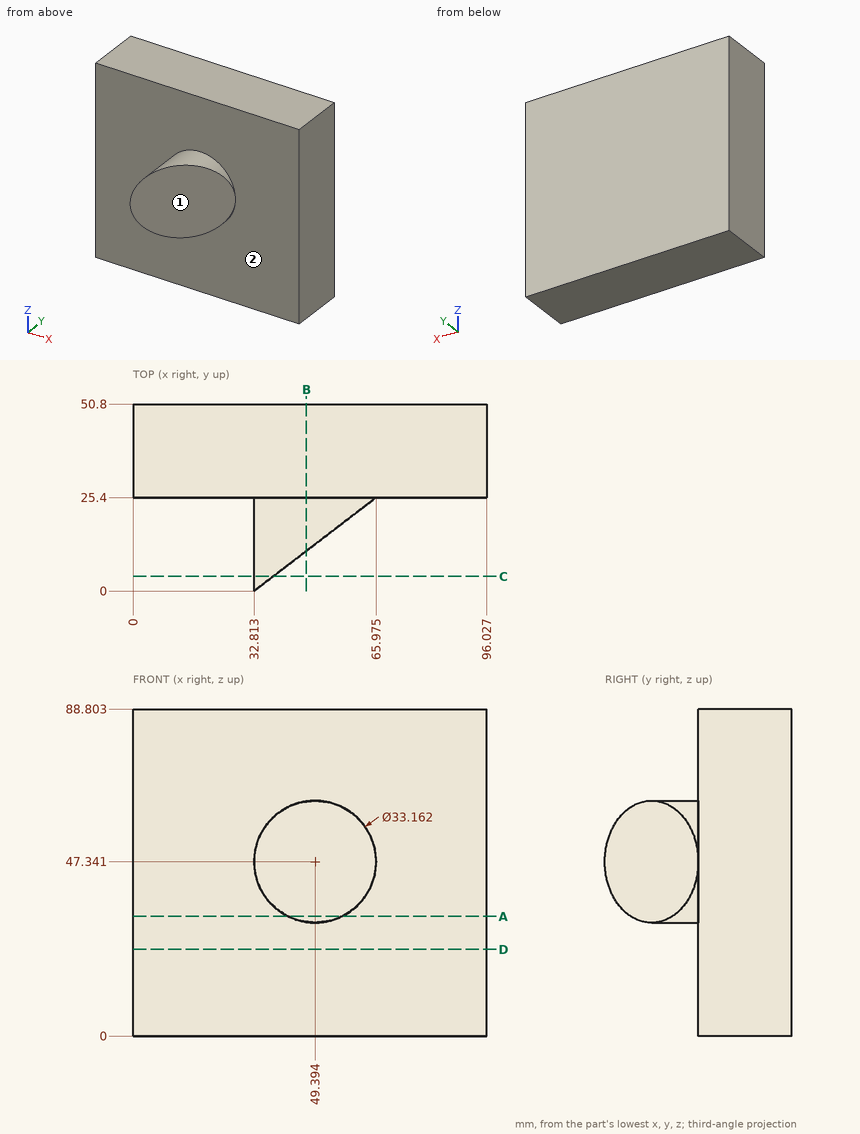
Source: three-view drawing plus pictorial views. Frame: mm from the lowest corner of the part. A direction names the side the tool comes from. Coordinates: 2 decimals unless noted, no trailing zeros. Order: outer loops, then holes, each group sorted by start corner. A loop starts at its lowest first (then second) coordinate and runs counter-clockwise, first axis right, second up.
Item 1: Material intervals for line 1 (Y direction, x = 26.5, z = 21.5); line 2 (X direction, y = 16, z = 46.5) (1 decimal); line 3 (Y direction, x = 54, z = 57), sorted ascending.
Output values:
line 1: y = 25.4 to 50.8
line 2: x = 32.8 to 53.7
line 3: y = 16.23 to 50.8
Item 2: Cut plane D-D (z = 23.5). Return loops of the section in (x, y), plus the area to 3 significant figures.
Output values:
outline: (0, 25.4) - (96.03, 25.4) - (96.03, 50.8) - (0, 50.8) - close
area: 2,440 mm2
Item 3: Cut plane B-B (x = 47). Return loops of the section in (y, z), plus the area to 3 significant figures.
Output values:
outline: (10.87, 30.93) - (25.4, 30.93) - (25.4, 0) - (50.8, 0) - (50.8, 88.8) - (25.4, 88.8) - (25.4, 63.75) - (10.87, 63.75) - close
area: 2,730 mm2
Item 4: Cut plane A-A (z = 32.5). Return loops of the section in (x, y), plus the area to 3 significant figures.
Output values:
outline: (0, 25.4) - (42, 25.4) - (42, 7.04) - (56.79, 18.36) - (56.79, 25.4) - (96.03, 25.4) - (96.03, 50.8) - (0, 50.8) - close
area: 2,630 mm2
Item 5: Set-up query: the marked faces 1 and 2. Return all of +Z, -Z, +X, -X, +Y, -Y with unobstructed straight access to the full face (end or side cutting, diameter ignored); none if empty.
Output values:
face 1: +Z, -Z, +X, -Y
face 2: -Y
Item 6: First-contact query: P1, Ø3, axis at x = 72.5, z = 46.5, coming from the -Y side; P2, Ø1, axis at y = 7, z = 62, coming from the -X side (1 decimal); P3, Ø4, axis at x = 42, z = 48, coming from the -Y side (1 decimal). Flat tips, straight axial feed; report the tip coordinate or a pass-through.
Output values:
P1: stops at y = 25.4
P2: stops at x = 40.8
P3: stops at y = 5.5
Item 7: Cut plane C-C (y = 4). Return loops of the section in (x, z) (1 decimal).
Output values:
outline: (38, 35.3) - (38, 59.4) arc R16.6 ccw to start
